Check sheet for the modelled part. Datum: model origin and axes. Units: mm. A direction names the side the tool comes from. Round coordinates to 2 decimals unless told otherwise and drop trailing zeros. Loops run counter-clockwise (first coordinate to the right, second up) from the corner with the lowest first, then second, coordinate; pieces in that order, holes last. Notation, with made-up numbers: (70.5, 54) - (95.5, 54) arc R21 ccw to (95.5, 89) - close; hole circle Ø2 at (-40, 89). An arc over 180 degrees is marked (long way). Put each result on its own line as item: value.
Autodesk Fusion 360 part; units mm, degrees
sketch "Sketch1" plane through (0, 0, 0) normal (0, 0, 1) x (1, 0, 0)
  circle A0 centre (0, 0) radius 6.15
  dimension "d1" = 12.3
ref_plane "WorkPlane1" through (0, 0, 10) normal (0, 0, 1) x (1, 0, 0)
sketch "Sketch2" plane through (0, 0, 10) normal (0, 0, 1) x (1, 0, 0)
  circle A0 centre (0, 0) radius 7.75
  dimension "d3" = 15.5
loft "Loft1" add profiles "Sketch2", "Sketch1" section 1 section 2
sketch "Sketch3" plane through (0, 0, 10) normal (0, 0, 1) x (1, 0, 0)
  circle A0 centre (0, 0) radius 7.75
  circle A1 centre (0, 0) radius 9.575
  dimension "d4" = 19.15
extrude "Extrude1" add sketch "Sketch3" along normal blind 6.5 contours A0 | A1
sketch "Sketch4" plane through (0, 0, 16.5) normal (0, 0, 1) x (1, 0, 0)
  circle A0 centre (0, 0) radius 9.575
  circle A1 centre (0, 0) radius 5.25 construction
  line L0 (0, 5.25) -> (0, -5.25) construction
  circle A2 centre (0, 5.25) radius 0.5
  circle A3 centre (-3.7123, 3.7123) radius 0.5
  circle A4 centre (-3.7123, -3.7123) radius 0.5
  circle A5 centre (0, -5.25) radius 0.5
  circle A6 centre (3.7123, -3.7123) radius 0.5
  circle A7 centre (3.7123, 3.7123) radius 0.5
  dimension "d7" = 10.5
  dimension "d8" = 1
  dimension "d10" = 360

Autodesk Fusion 360 part; units mm, degrees
sketch "Sketch1" plane through (0, 0, 0) normal (0, 0, 1) x (1, 0, 0)
  circle A0 centre (0, 0) radius 8.25
  dimension "d1" = 16.5
extrude "Extrude1" add sketch "Sketch1" along normal blind 11.5
Item 1: Tool access check on faces 1 (the flat face through (3, 8, 10)), 2 (the cylindrical face through (-7.598, 5.826, 13.204)). Record the directions out of +Z, -Z, +X, -X, +Y, -Y that give a thin tool (end or side, any length) a straight path to the whole face; none if there is none.
Filled sheet:
face 1: -Z
face 2: +Z, -Z
Item 2: Section check D-D on z = 13. Enter the section's corners in (x, y) (3 decimals).
Filled sheet:
outline: circle Ø19.15 at (0, 0)
Item 3: Section check A-A on x = 0. Enter the section's corners in (y, z) (3 decimals), then the cut area to 3 significant figures.
Filled sheet:
outline: (-9.575, 10) - (-8.25, 10) - (-8.25, 0) - (8.25, 0) - (8.25, 10) - (9.575, 10) - (9.575, 16.5) - (-9.575, 16.5) - close
area: 289 mm²
Item 4: Thickness scan on line 1 (Z direction, x = 7, y = -4.5); line 2 (Y direction, x = 0, z = 2.5); line 3 (X direction, y = -5.75, z = 6). Record the ranges inside material, lowest first. Write a range as from..to.
Filled sheet:
line 1: 10..16.5
line 2: -8.25..8.25
line 3: -5.92..5.92
Item 5: Section check C-C on z = 6.25. Enter the section's corners in (x, y), then the cut area to 3 significant figures.
Filled sheet:
outline: circle Ø16.5 at (0, 0)
area: 214 mm²
